Geometry check sheet. Reference: drawing and pictorial views, mm from the part's lowest x, y, z. A direction names the side the tool comes from. Give positions to 0.01 mm unless a question says otherwise; leave off trailing zeros. Write each loop counter-clockwise with the first axis right and the second up, starting at its lowest first coordinate (ties: lowest second). Pieces come first, ordered by that corner, then holes. Notation, with made-up numbers: M 71,66 L 92,66 A23 cw 92,86 Z; hole C 54.5,79.25 d4. An arc over 180 degrees is marked long. Answer as a JSON object with one key per item and string values.
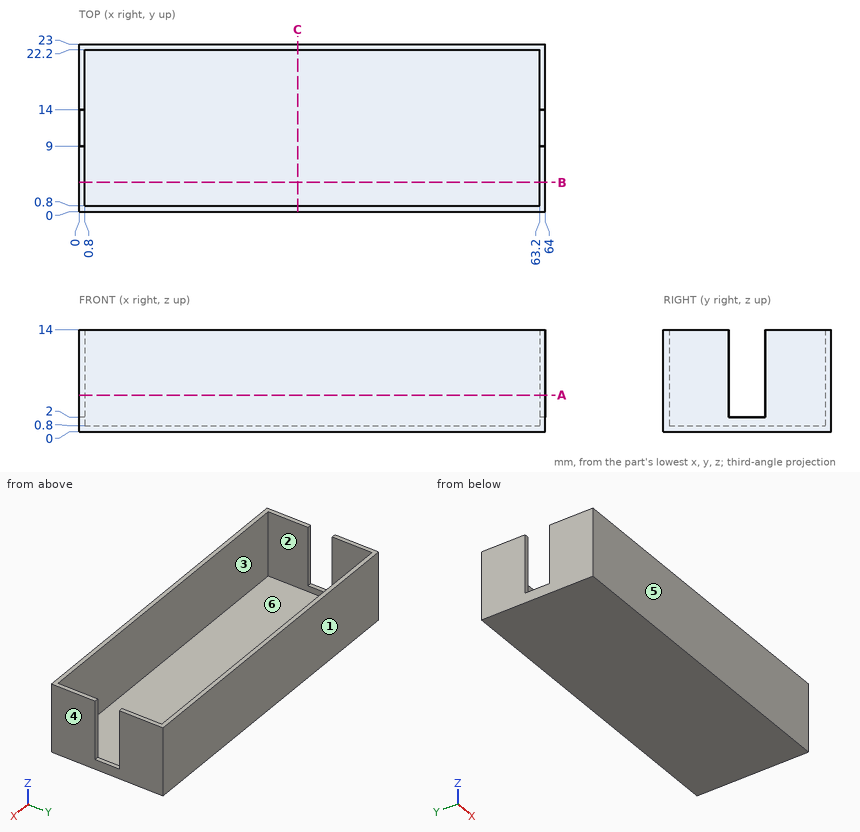
1) Section check C-C on x = 30. Record the boundary of the cut face in (y, z).
Completed:
{"outline": "M 0,0 L 23,0 L 23,14 L 22.2,14 L 22.2,0.8 L 0.8,0.8 L 0.8,14 L 0,14 Z"}
2) Release check for a two-part mould opening along X. For the marked faces 3, 4, 5 and 6 record: pulls with the +X half, pulls with the -X half, needs draft (parallel to the pull), parting line crosses it, or undercut.
Completed:
{"face 3": "undercut", "face 4": "pulls with the +X half", "face 5": "needs draft", "face 6": "undercut"}
3) Access from +Z, -Z, +X, -X, +Y, -Y to the whole of each face (thin tool, end or side, straight path). Record for the marked faces 1 and 2.
Completed:
{"face 1": "+Z, -Z, +X, -X, +Y", "face 2": "+Z"}
4) Thickness scan on L1, parallel to X at y = 1.75, z = 9.75; L2, parallel to Y at x = 8.5, z = 2.75; L3, parallel to Z at x = 42.5, y = 21.5. Record the ranges inside material, lowest first.
Completed:
{"L1": "x = 0 to 0.8, 63.2 to 64", "L2": "y = 0 to 0.8, 22.2 to 23", "L3": "z = 0 to 0.8"}
5) Section check B-B on y = 4. Record the boundary of the cut face in (x, z).
Completed:
{"outline": "M 0,0 L 64,0 L 64,14 L 63.2,14 L 63.2,0.8 L 0.8,0.8 L 0.8,14 L 0,14 Z"}
6) Go/stop test with flat-tipped pins: pin 1 (5 mm diameter, centred on y = 4, z = 12.5, fed in from -X); pin 2 (0.9 mm diameter, centred on x = 0, y = 11, fed in from +Z); pin 3 (6.5 mm diameter, centred on x = 26.5, y = 12, fed in from +Z). Record where each tip stops, or that it passes through.
Completed:
{"pin 1": "stops at x = 0", "pin 2": "stops at z = 2", "pin 3": "stops at z = 0.8"}
7) Section check A-A on z = 5. Record the boundary of the cut face in (x, y), and give its area (3 significant figures).
Completed:
{"outline": "M 0,0 L 64,0 L 64,9 L 63.2,9 L 63.2,0.8 L 0.8,0.8 L 0.8,9 L 0,9 Z; M 0,14 L 0.8,14 L 0.8,22.2 L 63.2,22.2 L 63.2,14 L 64,14 L 64,23 L 0,23 Z", "area": "129 mm2"}
